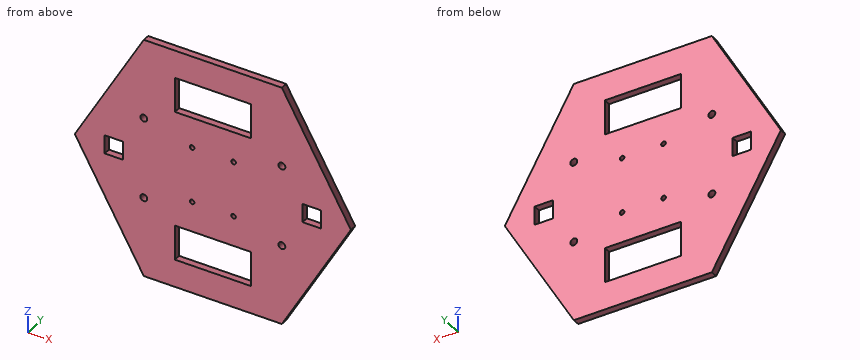
from build123d import *

# Parameters (mm, degrees)
SALIENTE_EXTRUIR1_DEPTH = 3
CROQUIS3_W              = 33
CROQUIS3_H              = 15
CORTAR_EXTRUIR1_DEPTH   = 4
CROQUIS4_R              = 1
CORTAR_EXTRUIR2_DEPTH   = 4
CROQUIS5_W              = 8
CROQUIS5_H              = 8
CORTAR_EXTRUIR3_DEPTH   = 4
CROQUIS6_R              = 1.5
CORTAR_EXTRUIR4_DEPTH   = 4


with BuildPart() as part:
    # Croquis1 → Saliente-Extruir1 (new body)
    with BuildSketch(Plane(origin=(0, 0, 0), x_dir=(1, 0, 0), z_dir=(0, 1, 0))):
        Polygon((-60, 0), (-30, -51.961524227), (30, -51.961524227), (60, 0), (30, 51.961524227), (-30, 51.961524227), align=None)
    extrude(amount=SALIENTE_EXTRUIR1_DEPTH)

    # Croquis3 → Cortar-Extruir1 (cut, through all)
    with BuildSketch(Plane(origin=(0, 3, 0), x_dir=(1, 0, 0), z_dir=(0, 1, 0))):
        with Locations((0, -32.5)):
            Rectangle(CROQUIS3_W, CROQUIS3_H)
        with Locations((0, 32.5)):
            Rectangle(CROQUIS3_W, CROQUIS3_H)
    extrude(amount=-CORTAR_EXTRUIR1_DEPTH, mode=Mode.SUBTRACT)

    # Croquis4 → Cortar-Extruir2 (cut, through all)
    with BuildSketch(Plane(origin=(0, 3, 0), x_dir=(1, 0, 0), z_dir=(0, 1, 0))):
        with Locations((-9, -11.95)):
            Circle(CROQUIS4_R)
        with Locations((9, -11.95)):
            Circle(CROQUIS4_R)
        with Locations((9, 11.95)):
            Circle(CROQUIS4_R)
        with Locations((-9, 11.95)):
            Circle(CROQUIS4_R)
    extrude(amount=-CORTAR_EXTRUIR2_DEPTH, mode=Mode.SUBTRACT)

    # Croquis5 → Cortar-Extruir3 (cut, through all)
    with BuildSketch(Plane(origin=(0, 3, 0), x_dir=(1, 0, 0), z_dir=(0, 1, 0))):
        with Locations((-43, 0)):
            Rectangle(CROQUIS5_W, CROQUIS5_H)
        with Locations((43, 0)):
            Rectangle(CROQUIS5_W, CROQUIS5_H)
    extrude(amount=-CORTAR_EXTRUIR3_DEPTH, mode=Mode.SUBTRACT)

    # Croquis6 → Cortar-Extruir4 (cut, through all)
    with BuildSketch(Plane(origin=(0, 3, 0), x_dir=(1, 0, 0), z_dir=(0, 1, 0))):
        with Locations((-30, -17.5)):
            Circle(CROQUIS6_R)
        with Locations((-30, 17.5)):
            Circle(CROQUIS6_R)
        with Locations((30, 17.5)):
            Circle(CROQUIS6_R)
        with Locations((30, -17.5)):
            Circle(CROQUIS6_R)
    extrude(amount=-CORTAR_EXTRUIR4_DEPTH, mode=Mode.SUBTRACT)


solid = part.part
Here's how the part is built. I have some questions about the finished solid (model axes, mm). Coordinates: 2 decimals unless noted, no trailing zeros. Order: outer loops, then holes, each group sorted by start corner. A loop starts at its lowest first (then second) coordinate and runs counter-clockwise, first axis right, second up.
Item 1: If we section it at B-B on z = 17.5: List the corners of the cut face in (x, y) for me, plus the area to 3 significant figures.
Result sheet:
outline: (-49.9, 0) - (-31.5, 0) - (-31.5, 3) - (-49.9, 3) - close; (-28.5, 0) - (28.5, 0) - (28.5, 3) - (-28.5, 3) - close; (31.5, 0) - (49.9, 0) - (49.9, 3) - (31.5, 3) - close
area: 281 mm2
Item 2: For P1, Ø1.5, axis at x = -43.5, y = 1, coming from the -Z side; P2, Ø10, axis at x = 34.5, z = 32.5, coming from the -Y side; P3, Ø1.5, axis at x = -41, y = 2.5, coming from the -Z side; P4, Ø0.9, axis at y = 1.5, z = -30, coming from the -X side, each with a flat end and sliding along its axis, tell me the tip position at first contact or that it passes through.
Result sheet:
P1: stops at z = -29.88
P2: stops at y = 0
P3: stops at z = -34.21
P4: stops at x = -42.94
Item 3: I need wall thicknesses on line 1 (Z direction, x = -11.5, y = 2.1); line 2 (Z direction, x = 9, y = 1.1); line 3 (Z direction, x = -30, y = 1.4). Which ranges of each line are inside material? Lowest first, please.
Result sheet:
line 1: z = -51.96 to -40, -25 to 25, 40 to 51.96
line 2: z = -51.96 to -40, -25 to -12.95, -10.95 to 10.95, 12.95 to 25, 40 to 51.96
line 3: z = -51.96 to -19, -16 to 16, 19 to 51.96
Item 4: If we section it at A-A on y = 1.9: State how many separate pieces and enclosed holes the cut face has, plus the area to 3 significant figures.
Result sheet:
separate pieces: 1
enclosed holes: 12
area: 8,190 mm2
Item 5: If we section it at C-C on x = 40.5: List the corners of the cut face in (y, z) for me (3 decimals), plus the area to 3 significant figures.
Result sheet:
outline: (0, -33.775) - (3, -33.775) - (3, -4) - (0, -4) - close; (0, 4) - (3, 4) - (3, 33.775) - (0, 33.775) - close
area: 179 mm2
Item 6: If we section it at D-D on z = -36: List the corners of the cut face in (x, y) for me, plus the area to 3 significant figures.
Result sheet:
outline: (-39.22, 0) - (-16.5, 0) - (-16.5, 3) - (-39.22, 3) - close; (16.5, 0) - (39.22, 0) - (39.22, 3) - (16.5, 3) - close
area: 136 mm2
